from build123d import *

# Parameters (mm, degrees)
F0_R     = 2.5
F1_DEPTH = 500


with BuildPart() as f1:
    # F0 (on Top) → F1 (new body)
    with BuildSketch(Plane.XY):
        with BuildLine():
            Line((-0.206975, 13.902523), (-2.845819, 13.902523))
            Line((-2.845819, 13.902523), (-5.497237, 16.55394))
            Line((-5.497237, 16.55394), (-5.497237, 18.202523))
            Line((-5.497237, 18.202523), (-2.885113, 18.202523))
            Line((-2.885113, 18.202523), (-2.885113, 18.30915))
            Line((-2.885113, 18.30915), (-4.400227, 19.824264))
            ThreePointArc((-4.400227, 19.824264), (-4.594881, 19.954328), (-4.824491, 20))
            Line((-4.824491, 20), (-8.5, 20))
            ThreePointArc((-8.5, 20), (-9.074025, 19.885819), (-9.56066, 19.56066))
            ThreePointArc((-9.56066, 19.56066), (-9.885819, 19.074025), (-10, 18.5))
            Line((-10, 18.5), (-10, 14.824491))
            ThreePointArc((-10, 14.824491), (-9.954328, 14.594881), (-9.824264, 14.400227))
            Line((-9.824264, 14.400227), (-8.30915, 12.885113))
            Line((-8.30915, 12.885113), (-8.202523, 12.885113))
            Line((-8.202523, 12.885113), (-8.202523, 15.497237))
            Line((-8.202523, 15.497237), (-6.55394, 15.497237))
            Line((-6.55394, 15.497237), (-3.902523, 12.845819))
            Line((-3.902523, 12.845819), (-3.902523, 10.206975))
            Line((-3.902523, 10.206975), (-3.695548, 10))
            Line((-3.695548, 10), (-3.902523, 9.793025))
            Line((-3.902523, 9.793025), (-3.902523, 7.154181))
            Line((-3.902523, 7.154181), (-6.55394, 4.502763))
            Line((-6.55394, 4.502763), (-8.202523, 4.502763))
            Line((-8.202523, 4.502763), (-8.202523, 7.114887))
            Line((-8.202523, 7.114887), (-8.30915, 7.114887))
            Line((-8.30915, 7.114887), (-9.824264, 5.599773))
            ThreePointArc((-9.824264, 5.599773), (-9.954328, 5.405119), (-10, 5.175509))
            Line((-10, 5.175509), (-10, 0))
            Line((-10, 0), (-10, -5.175509))
            ThreePointArc((-10, -5.175509), (-9.954328, -5.405119), (-9.824264, -5.599773))
            Line((-9.824264, -5.599773), (-8.30915, -7.114887))
            Line((-8.30915, -7.114887), (-8.202523, -7.114887))
            Line((-8.202523, -7.114887), (-8.202523, -4.502763))
            Line((-8.202523, -4.502763), (-6.55394, -4.502763))
            Line((-6.55394, -4.502763), (-3.902523, -7.154181))
            Line((-3.902523, -7.154181), (-3.902523, -9.793025))
            Line((-3.902523, -9.793025), (-3.695548, -10))
            Line((-3.695548, -10), (-3.902523, -10.206975))
            Line((-3.902523, -10.206975), (-3.902523, -12.845819))
            Line((-3.902523, -12.845819), (-6.55394, -15.497237))
            Line((-6.55394, -15.497237), (-8.202523, -15.497237))
            Line((-8.202523, -15.497237), (-8.202523, -12.885113))
            Line((-8.202523, -12.885113), (-8.30915, -12.885113))
            Line((-8.30915, -12.885113), (-9.824264, -14.400227))
            ThreePointArc((-9.824264, -14.400227), (-9.954328, -14.594881), (-10, -14.824491))
            Line((-10, -14.824491), (-10, -18.5))
            ThreePointArc((-10, -18.5), (-9.885819, -19.074025), (-9.56066, -19.56066))
            ThreePointArc((-9.56066, -19.56066), (-9.074025, -19.885819), (-8.5, -20))
            Line((-8.5, -20), (-4.824491, -20))
            ThreePointArc((-4.824491, -20), (-4.594881, -19.954328), (-4.400227, -19.824264))
            Line((-4.400227, -19.824264), (-2.885113, -18.30915))
            Line((-2.885113, -18.30915), (-2.885113, -18.202523))
            Line((-2.885113, -18.202523), (-5.497237, -18.202523))
            Line((-5.497237, -18.202523), (-5.497237, -16.55394))
            Line((-5.497237, -16.55394), (-2.845819, -13.902523))
            Line((-2.845819, -13.902523), (-0.206975, -13.902523))
            Line((-0.206975, -13.902523), (0, -13.695548))
            Line((0, -13.695548), (0.206975, -13.902523))
            Line((0.206975, -13.902523), (2.845819, -13.902523))
            Line((2.845819, -13.902523), (5.497237, -16.55394))
            Line((5.497237, -16.55394), (5.497237, -18.202523))
            Line((5.497237, -18.202523), (2.885113, -18.202523))
            Line((2.885113, -18.202523), (2.885113, -18.30915))
            Line((2.885113, -18.30915), (4.400227, -19.824264))
            ThreePointArc((4.400227, -19.824264), (4.594881, -19.954328), (4.824491, -20))
            Line((4.824491, -20), (8.5, -20))
            ThreePointArc((8.5, -20), (9.074025, -19.885819), (9.56066, -19.56066))
            ThreePointArc((9.56066, -19.56066), (9.885819, -19.074025), (10, -18.5))
            Line((10, -18.5), (10, -14.824491))
            ThreePointArc((10, -14.824491), (9.954328, -14.594881), (9.824264, -14.400227))
            Line((9.824264, -14.400227), (8.30915, -12.885113))
            Line((8.30915, -12.885113), (8.202523, -12.885113))
            Line((8.202523, -12.885113), (8.202523, -15.497237))
            Line((8.202523, -15.497237), (6.55394, -15.497237))
            Line((6.55394, -15.497237), (3.902523, -12.845819))
            Line((3.902523, -12.845819), (3.902523, -10.206975))
            Line((3.902523, -10.206975), (3.695548, -10))
            Line((3.695548, -10), (3.902523, -9.793025))
            Line((3.902523, -9.793025), (3.902523, -7.154181))
            Line((3.902523, -7.154181), (6.55394, -4.502763))
            Line((6.55394, -4.502763), (8.202523, -4.502763))
            Line((8.202523, -4.502763), (8.202523, -7.114887))
            Line((8.202523, -7.114887), (8.30915, -7.114887))
            Line((8.30915, -7.114887), (9.824264, -5.599773))
            ThreePointArc((9.824264, -5.599773), (9.954328, -5.405119), (10, -5.175509))
            Line((10, -5.175509), (10, 0))
            Line((10, 0), (10, 5.175509))
            ThreePointArc((10, 5.175509), (9.954328, 5.405119), (9.824264, 5.599773))
            Line((9.824264, 5.599773), (8.30915, 7.114887))
            Line((8.30915, 7.114887), (8.202523, 7.114887))
            Line((8.202523, 7.114887), (8.202523, 4.502763))
            Line((8.202523, 4.502763), (6.55394, 4.502763))
            Line((6.55394, 4.502763), (3.902523, 7.154181))
            Line((3.902523, 7.154181), (3.902523, 9.793025))
            Line((3.902523, 9.793025), (3.695548, 10))
            Line((3.695548, 10), (3.902523, 10.206975))
            Line((3.902523, 10.206975), (3.902523, 12.845819))
            Line((3.902523, 12.845819), (6.55394, 15.497237))
            Line((6.55394, 15.497237), (8.202523, 15.497237))
            Line((8.202523, 15.497237), (8.202523, 12.885113))
            Line((8.202523, 12.885113), (8.30915, 12.885113))
            Line((8.30915, 12.885113), (9.824264, 14.400227))
            ThreePointArc((9.824264, 14.400227), (9.954328, 14.594881), (10, 14.824491))
            Line((10, 14.824491), (10, 18.5))
            ThreePointArc((10, 18.5), (9.885819, 19.074025), (9.56066, 19.56066))
            ThreePointArc((9.56066, 19.56066), (9.074025, 19.885819), (8.5, 20))
            Line((8.5, 20), (4.824491, 20))
            ThreePointArc((4.824491, 20), (4.594881, 19.954328), (4.400227, 19.824264))
            Line((4.400227, 19.824264), (2.885113, 18.30915))
            Line((2.885113, 18.30915), (2.885113, 18.202523))
            Line((2.885113, 18.202523), (5.497237, 18.202523))
            Line((5.497237, 18.202523), (5.497237, 16.55394))
            Line((5.497237, 16.55394), (2.845819, 13.902523))
            Line((2.845819, 13.902523), (0.206975, 13.902523))
            Line((0.206975, 13.902523), (0, 13.695548))
            Line((0, 13.695548), (-0.206975, 13.902523))
        make_face()
        Polygon((-7.11684, -17.11684), (-6.573574, -17.660106), (-6.573574, -18.202523), (-8.202523, -18.202523), (-8.202523, -16.573574), (-7.660106, -16.573574), align=None, mode=Mode.SUBTRACT)
        Polygon((7.11684, -17.11684), (7.660106, -16.573574), (8.202523, -16.573574), (8.202523, -18.202523), (6.573574, -18.202523), (6.573574, -17.660106), align=None, mode=Mode.SUBTRACT)
        with Locations((0, -10)):
            Circle(F0_R, mode=Mode.SUBTRACT)
        Polygon((-6.573574, 18.202523), (-6.573574, 17.660106), (-7.11684, 17.11684), (-7.660106, 16.573574), (-8.202523, 16.573574), (-8.202523, 18.202523), align=None, mode=Mode.SUBTRACT)
        Polygon((0.206975, 6.097477), (2.845819, 6.097477), (6.240773, 2.702523), (8.199174, 2.702523), (8.199174, 0), (8.199174, -2.702523), (6.240773, -2.702523), (2.845819, -6.097477), (0.206975, -6.097477), (0, -6.304452), (-0.206975, -6.097477), (-2.845819, -6.097477), (-6.240773, -2.702523), (-8.199174, -2.702523), (-8.199174, 0), (-8.199174, 2.702523), (-6.240773, 2.702523), (-2.845819, 6.097477), (-0.206975, 6.097477), (0, 6.304452), align=None, mode=Mode.SUBTRACT)
        with Locations((0, 10)):
            Circle(F0_R, mode=Mode.SUBTRACT)
        Polygon((7.11684, 17.11684), (6.573574, 17.660106), (6.573574, 18.202523), (8.202523, 18.202523), (8.202523, 16.573574), (7.660106, 16.573574), align=None, mode=Mode.SUBTRACT)
    extrude(amount=F1_DEPTH)


solid = f1.part
Work out the finished part from the listing and answer in its coordinate system (mm). Coordinates: 2 decimals unless noted, no trailing zeros. Put each result on its own line as item: value. Start each with the question number.
1) Flat-ended cylindrical pins translate along their axes: pin 1 (2 mm diameter, centred on y = -8.5, z = 161, fed in from -X); pin 2 (0.8 mm diameter, centred on y = 8.5, z = 141, fed in from +X). Find the tip coordinate at first contact, or state that the pin passes through.
2) Find the intervals of material crossed by line 1 (Y direction, x = 0, z = 267.5); line 2 (Y direction, x = 0.5, z = 242); line 3 (X direction, y = 10.5, z = 346), in increasing order. Write a range as from..to.
3) Find section A-A (z = 228.5). State how many separate pieces and enclosed holes the cut face has, plus the area to 3 significant figures.
Results list:
1. pin 1: stops at x = -3.9
1. pin 2: stops at x = 3.9
2. line 1: y = -13.7..-12.5, -7.5..-6.3, 6.3..7.5, 12.5..13.7
2. line 2: y = -13.9..-12.45, -7.55..-6.1, 6.1..7.55, 12.45..13.9
2. line 3: x = -3.9..-2.45, 2.45..3.9
3. separate pieces: 1
3. enclosed holes: 7
3. area: 279 mm^2
